The listing builds one solid part. Answer for the finished solid, in the listing's coordinates (mm). Face numbers are marked on the shaded views. Give positions to 0.01 mm unless a question says otherwise; leave off trailing zeros. Write each loop counter-clockwise with the first axis right and the second up, starting at its lowest first coordinate (ties: lowest second). Pieces come first, ordered by that corner, then holes. Notation, with made-up numbers: (46.25, 47) -> (104.25, 47) arc R29 ccw to (104.25, 81) -> close; hole circle Ø2 at (48, 24). An arc over 180 degrees is marked (long way). Put each result on its own line as item: value. Start each with the question number.
1) A cutting plane is placed at B-B (y = -207.5). Write down the section's boundary in (x, z) (3 decimals), then the cut area to 3 significant figures.
2) Find the intervals of material crossed by line 1 along Y through (x, z) = (-47, -22.5) (3 decimals); line 2 along Y through (x, z) = (-1099.5, -5.5); line 3 along X through (y, z) = (171.5, -14) (3 decimals), in increasing order. Write a range as from..to.
3) A cutting plane is placed at D-D (y = -398). Write down the section's boundary in (x, z) (3 decimals).
4) Flat-ended cylindrical pins translate along their axes: pin 1 Ø1.5 at (y, z) = (-32, -3.5) entering from +X; pin 2 Ø15 at (x, z) = (555.5, -13.5) entering from +Y; pin 3 Ø1 at (y, z) = (25, -1) entering from -X; pin 4 Ø8 at (x, z) = (31.5, -2.5) entering from -Y. Find the tip coordinate at first contact, or state that the pin passes through.
5) For a pull along X with two mould halves and no side action, classify the marked faces 1 and 2 as released by +X, released by -X, zero draft, split by the parting line, or undercut.
6) A cutting plane is placed at C-C (x = 453.5). Write down the section's boundary in (y, z) (3 decimals), then the cut area to 3 significant figures.
7) A cutting plane is placed at A-A (z = -11.5). Write down the section's boundary in (x, y) (3 decimals).
from build123d import *

# Parameters (mm, degrees)
F0_W     = 2692.4
F0_H     = 914.4
F1_DEPTH = 3.175


with BuildPart() as f1:
    # F0 (on Top) → F1 (new body)
    with BuildSketch(Plane.XY):
        Rectangle(F0_W, F0_H)
    extrude(amount=F1_DEPTH)

    # F4: sweep along a path in F2
    with BuildLine(Plane(origin=(0, 0, 0), x_dir=(1, 0, 0), z_dir=(0, 0, -1))) as f4_path:
        Line((-1295.4, 247.65), (-1295.4, -247.65))
        Line((-1295.4, -247.65), (1295.4, -247.65))
        Line((1295.4, -247.65), (1295.4, 247.65))
        Line((1295.4, 247.65), (-1295.4, 247.65))
    # F3 (on Front) → F4 (sweep)
    with BuildSketch(Plane.XZ):
        with BuildLine():
            Line((-1295.4, -25.4), (-1295.4, 0))
            Line((-1295.4, 0), (-1320.8, 0))
            Line((-1320.8, 0), (-1320.8, -3.175))
            Line((-1320.8, -3.175), (-1301.75, -3.175))
            ThreePointArc((-1301.75, -3.175), (-1299.5049359697, -4.1049359697), (-1298.575, -6.35))
            Line((-1298.575, -6.35), (-1298.575, -25.4))
            Line((-1298.575, -25.4), (-1295.4, -25.4))
        make_face()
    sweep(path=f4_path.line, transition=Transition.RIGHT)


solid = f1.part
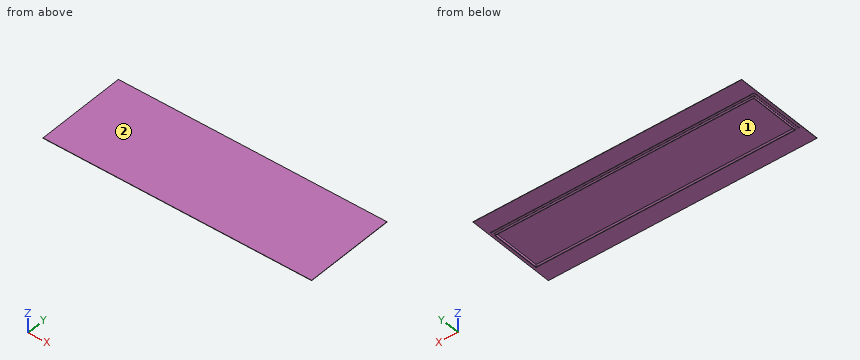
Reply:
1. outline: (-1346.2, 0) -> (-1320.8, 0) -> (-1320.8, -3.175) -> (-1301.75, -3.175) arc R3.175 cw to (-1298.575, -6.35) -> (-1298.575, -25.4) -> (-1295.4, -25.4) -> (-1295.4, 0) -> (1295.4, 0) -> (1295.4, -25.4) -> (1298.575, -25.4) -> (1298.575, -6.35) arc R3.175 cw to (1301.75, -3.175) -> (1320.8, -3.175) -> (1320.8, 0) -> (1346.2, 0) -> (1346.2, 3.175) -> (-1346.2, 3.175) -> close
1. area: 8,860 mm2
2. line 1: y = -250.825..-247.65, 247.65..250.825
2. line 2: y = -250.94..-247.65, 247.65..250.94
2. line 3: x = -1298.575..-1295.4, 1295.4..1298.575
3. outline: (-1346.2, 0) -> (1346.2, 0) -> (1346.2, 3.175) -> (-1346.2, 3.175) -> close
4. pin 1: stops at x = 1320.8
4. pin 2: stops at y = 250.84
4. pin 3: stops at x = -1320.8
4. pin 4: stops at y = -457.2
5. face 1: undercut
5. face 2: zero draft
6. outline: (-457.2, 0) -> (-273.05, 0) -> (-273.05, -3.175) -> (-254, -3.175) arc R3.175 cw to (-250.825, -6.35) -> (-250.825, -25.4) -> (-247.65, -25.4) -> (-247.65, 0) -> (247.65, 0) -> (247.65, -25.4) -> (250.825, -25.4) -> (250.825, -6.35) arc R3.175 cw to (254, -3.175) -> (273.05, -3.175) -> (273.05, 0) -> (457.2, 0) -> (457.2, 3.175) -> (-457.2, 3.175) -> close
6. area: 3,210 mm2
7. outline: (-1298.575, -250.825) -> (1298.575, -250.825) -> (1298.575, 250.825) -> (-1298.575, 250.825) -> close; hole (-1295.4, -247.65) -> (1295.4, -247.65) -> (1295.4, 247.65) -> (-1295.4, 247.65) -> close
